The listing builds one solid part. Answer for the finished solid, in the listing's coordinates (mm). A direction names the side the tool comes from. Round coordinates to 2 decimals unless told otherwise and drop trailing zeros. Order: outer loops, then holes, each group sorted by start corner. A loop starts at its lowest first (then second) coordinate and runs counter-clockwise, first axis right, second up. Notation, with made-up numbers: (13.5, 59) -> (27.5, 59) arc R15 ccw to (27.5, 69) -> close; hole circle Ø5 at (30.25, 1). An arc over 180 degrees is marked (long way). Return JSON: item names as keys, results as strings. Group by question number.
(1) The part is cut by section A-A (x = 0). Determine the outline of the cut face in (y, z), plus the area to 3 significant figures.
(2) The part is cut by section C-C (x = 8). Determine the outline of the cut face in (y, z), plus the area to 3 significant figures.
(3) Each of these flat-tipped pins is pushed along its axis until it touches: pin 1 (6 mm diameter, centred on x = 0, y = 6, fed in from -Z) (3 decimals); pin 2 (2 mm diameter, centred on x = 11.5, y = 14.5, fed in from -Z); pin 3 (2 mm diameter, centred on x = -9, y = 16, fed in from +Z). Where does it stop, or does it pass through?
(4) Which of the six approach directions +Z, -Z, +X, -X, +Y, -Y give full straight-line access (tool end or side, diameter ignored) to faces 1 (the face through (4.06, 5.03, -30.96)), 2 (the face through (6.552, 4.971, 29.506))?
(5) The part is cut by section B-B (y = 25.25). Determine the outline of the cut face in (x, z), plus the area to 3 significant figures.
(6) Consider line 1 (Z direction, x = 0, y = 5.5); line 2 (Z direction, x = -1, y = 19.25); line 3 (X direction, y = 6.75, z = 24). Determine where each line is inside the solid, lowest interval first. Write a range as [from, to].
from build123d import *

# Parameters (mm, degrees)
SKETCH_7_W               = 31.224989992
SKETCH_7_H               = 4
SHELL_2_T                = -1
CUT_EXTRUDE_4_DEPTH      = 55.534392818
CUT_EXTRUDE_4_DEPTH_BACK = 55.534392818


with BuildPart() as part:
    # 草图7 → 旋转12 (revolve)
    with BuildSketch(Plane.XY, mode=Mode.PRIVATE) as revolve_12_sk:
        with BuildLine():
            ThreePointArc((31.224989992, 7), (20, 24.979991994), (0, 32))
            Line((0, 32), (0, 7))
            Line((0, 7), (31.224989992, 7))
        make_face()
        with Locations((15.612494996, 5)):
            Rectangle(SKETCH_7_W, SKETCH_7_H)
    revolve(revolve_12_sk.sketch.rotate(Axis((0, 32, 0), (0, -1, 0)), 180), axis=Axis((0, 32, 0), (0, -1, 0)))

    # 抽壳2
    shell_2_openings = [part.faces().sort_by_distance(p)[0] for p in [
        (0, 3, 0),
    ]]
    offset(amount=SHELL_2_T, openings=shell_2_openings, kind=Kind.INTERSECTION)

    # 草图9 → 切除-拉伸4 (cut, two sides: drawn at the far end of the back side and taken through both)
    with BuildSketch(Plane.XY.offset(-CUT_EXTRUDE_4_DEPTH_BACK)):
        with BuildLine():
            ThreePointArc((-6.007581703, 31.431019107), (-13.478809235, 15.768247098), (-30.113359103, 10.825229952))
            ThreePointArc((-30.113359103, 10.825229952), (-20.792552221, 24.324263034), (-6.007581703, 31.431019107))
        make_face()
        with BuildLine():
            ThreePointArc((30.113359103, 10.825229952), (20.792552221, 24.324263034), (6.007581703, 31.431019107))
            ThreePointArc((6.007581703, 31.431019107), (13.478809235, 15.768247098), (30.113359103, 10.825229952))
        make_face()
    extrude(amount=CUT_EXTRUDE_4_DEPTH + CUT_EXTRUDE_4_DEPTH_BACK, mode=Mode.SUBTRACT)


solid = part.part
Answer below:
{
 "1": {"outline": "(3, -31.22) -> (7, -31.22) arc R32 ccw to (7, 31.22) -> (3, 31.22) -> (3, 30.22) -> (6.89, 30.22) arc R31 cw to (6.89, -30.22) -> (3, -30.22) -> close", "area": "92.8 mm²"},
 "2": {"outline": "(3, -30.18) -> (7, -30.18) arc R30.98 ccw to (22.98, -20.79) -> (22.98, -19.21) arc R29.95 cw to (6.89, -29.15) -> (3, -29.15) -> close; (3, 29.15) -> (6.89, 29.15) arc R29.95 cw to (22.98, 19.21) -> (22.98, 20.79) arc R30.98 ccw to (7, 30.18) -> (3, 30.18) -> close", "area": "47.5 mm²"},
 "3": {"pin 1": "stops at z = -31.225", "pin 2": "stops at z = -26.79", "pin 3": "stops at z = 26.88"},
 "4": {"face 1": "+Y, -Y", "face 2": "-Y"},
 "5": {"outline": "(-7.09, -18.33) arc R19.66 ccw to (7.09, -18.33) -> (7.09, -16.53) arc R17.98 cw to (-7.09, -16.53) -> close; (-7.09, 16.53) arc R17.98 cw to (7.09, 16.53) -> (7.09, 18.33) arc R19.66 ccw to (-7.09, 18.33) -> close", "area": "48.7 mm²"},
 "6": {"line 1": "z = [-31.22, -30.22], [30.22, 31.22]", "line 2": "z = [-25.54, -24.28], [24.28, 25.54]", "line 3": "x = [-19.97, -18.37], [18.37, 19.97]"}
}
